For this review, take the finished solid that the model builds, in its own axes (mm). A direction names the side the tool comes from. Give positions to 0.01 mm unless a question says otherwise; leave off trailing zeros. Loops run counter-clockwise (first coordinate to the right, second up) from the corner with the lowest first, then second, coordinate; pieces in that order, holes last.
```python
from build123d import *

# Parameters (mm, degrees)
F0_W     = 71.3519603014
F0_H     = 37.1488952078
F1_DEPTH = 40
F3_DEPTH = 25
F4_DEPTH = 12.1498952078
F5_T     = -2.5
F6_R     = 5


with BuildPart() as f1:
    # F0 (on Top) → F1 (new body)
    with BuildSketch(Plane.XY):
        with Locations((-16.4616554976, 14.1063730698)):
            Rectangle(F0_W, F0_H)
    extrude(amount=F1_DEPTH)

    # F2 (on face) → F3 (cut)
    with BuildSketch(Plane.XZ.offset(4.4680745341)):
        Polygon((-52.1376356483, 40), (-52.1376356483, 0), (19.2143246531, 40), align=None)
    extrude(amount=-F3_DEPTH, mode=Mode.SUBTRACT)

    # F4 (cut, through all): a face of the model
    f4_faces = [f1.faces().sort_by_distance(p)[0] for p in [
        (-28.3536488811, 20.5319254659, 26.6666666667),
    ]]
    extrude(f4_faces, amount=-F4_DEPTH, mode=Mode.SUBTRACT)

    # F5
    f5_openings = [f1.faces().sort_by_distance(p)[0] for p in [
        (19.214325, 14.106373, 20),
    ]]
    offset(amount=F5_T, openings=f5_openings)

    # F6
    f6_edges = [f1.edges().sort_by_distance(p)[0] for p in [
        (-16.461655, 32.680821, 20),
        (-16.461655, 32.680821, 0),
        (-16.461655, -4.468075, 20),
        (-16.461655, -4.468075, 0),
    ]]
    fillet(f6_edges, radius=F6_R)


solid = f1.part
```
Q1. Mouldability with a two-part tool opening along Z and no side actions: class faces 1 (the flat face through (19.214, -3, 20)), 2 (the flat face through (-17, 13.9, 19.7)), 3 (the flat face through (2, -1.968, 12)), 4 (the flat face through (-17, 14, 0)) as +Z half, -Z half, draft (parallel to the pull), parting line (faces both ways), or undercut.
Answers:
face 1: draft
face 2: +Z half
face 3: undercut
face 4: -Z half
Q2. Machinability: for faces 5 (the cylindrical face through (-15.962, -2.965, 1.426)), 6 (the flat face through (-12.108, 13.881, 19.575)), which of the approach directions +Z, -Z, +X, -X, +Y, -Y give a long, thin tool a straight path to every point of the face, cutting with its end or side? Answer none if there is none.
Answers:
face 5: -Z, +X, -X, -Y
face 6: +X
Q3. Consider section A-A on y = 7. Give the boundary of the cut face in (x, z), plus the area to 3 significant figures.
Answers:
outline: (-52.14, 0) - (19.21, 0) - (19.21, 2.5) - (-42.57, 2.5) - (19.21, 37.13) - (19.21, 40) - close
area: 357 mm2
Q4. For pin 1 Ø1 at (x, y) = (-9.5, 0.5) entering from +Z; pin 2 Ø4 at (y, z) = (7.5, 20) entering from +X; pin 3 Ø10 at (y, z) = (9, 8) entering from +X, all flat-tipped, find the tip position at first contact; note any pin that passes through.
Answers:
pin 1: stops at z = 24.18
pin 2: stops at x = -7.78
pin 3: stops at x = -23.84
Q5. For probe 1 along Y at (x, z) = (2, 25); probe 2 along Z at (x, y) = (13, 23); probe 3 along Y at (x, z) = (-4, 22), list the stretches that pass through material, from the lowest coordinate up.
Answers:
probe 1: y = -4.46 to -1.97, 30.18 to 32.67
probe 2: z = 0 to 2.5, 33.65 to 36.52
probe 3: y = -4.43 to -1.97, 30.18 to 32.64
